Check sheet for the modelled part. Datum: model origin and axes. Units: mm. A direction names the side the tool comes from. Round coordinates to 2 decimals unless told otherwise and drop trailing zeros. Write each loop counter-clockwise with the first axis right and the second up, starting at its lowest first coordinate (ties: lowest second). Pieces come first, ordered by that corner, then holes. Notation, with made-up numbers: M 11.25,22 L 29.25,22 A18 ccw 29.25,53 Z; hole C 39.5,42 d10. An arc over 180 degrees is marked long. Answer in a Markdown table with one row per item.
```python
from build123d import *

# Parameters (mm, degrees)
SKETCH1_R           = 3.875
BOSS_EXTRUDE1_DEPTH = 29.78
SKETCH2_OUTSIDE_W   = 16.096
SKETCH2_OUTSIDE_H   = 16.096
SKETCH2_OUTSIDE_R   = 2.39
CUT_EXTRUDE1_DEPTH  = 25
CHAMFER1_SIZE       = 0.5
CUT_EXTRUDE2_DEPTH  = 3.36


with BuildPart() as part:
    # Sketch1 → Boss-Extrude1 (new body)
    with BuildSketch(Plane(origin=(0, 0, 0), x_dir=(1, 0, 0), z_dir=(0, 1, 0))):
        Circle(SKETCH1_R)
    extrude(amount=BOSS_EXTRUDE1_DEPTH)

    # Sketch2 outside → Cut-Extrude1 (cut)
    with BuildSketch(Plane(origin=(0, 29.78, 0), x_dir=(1, 0, 0), z_dir=(0, 1, 0))):
        Rectangle(SKETCH2_OUTSIDE_W, SKETCH2_OUTSIDE_H)
        Circle(SKETCH2_OUTSIDE_R, mode=Mode.SUBTRACT)
    extrude(amount=-CUT_EXTRUDE1_DEPTH, mode=Mode.SUBTRACT)

    # Chamfer1
    chamfer1_edges = [part.edges().sort_by_distance(p)[0] for p in [
        (-2.39, 29.78, 0),
    ]]
    chamfer(chamfer1_edges, length=CHAMFER1_SIZE)

    # Sketch8 → Cut-Extrude2 (cut)
    with BuildSketch(Plane.XZ):
        Polygon((2.644264233, 0), (1.322132116, 2.29), (-1.322132116, 2.29), (-2.644264233, 0), (-1.322132116, -2.29), (1.322132116, -2.29), align=None)
    extrude(amount=-CUT_EXTRUDE2_DEPTH, mode=Mode.SUBTRACT)


solid = part.part
```
1. Scan lines: L1, parallel to Y at x = -2.75, z = 0.25; L2, parallel to Z at x = 0, y = 14.25; L3, parallel to X at y = 2.5, z = 0.5. Record each from-to range of solid material in increasing order.
Found:
| item | result |
|---|---|
| L1 | y = 0 to 4.78 |
| L2 | z = -2.39 to 2.39 |
| L3 | x = -3.84 to -2.36, 2.36 to 3.84 |
2. Section check C-C, the plane z = 3.5. Record the cut outline in (x, y).
Found:
| item | result |
|---|---|
| outline | M -1.66,0 L 1.66,0 L 1.66,4.78 L -1.66,4.78 Z |
3. Access from +Z, -Z, +X, -X, +Y, -Y to the whole of each face (thin tool, end or side, straight path). Record for faces 1 (the face through (-2, 0, 2)), 2 (the face through (1.974, 1.656, -1.161)), 3 (the face through (-2, 4.78, 2)).
Found:
| item | result |
|---|---|
| face 1 | +Z, -Z, +X, -X, -Y |
| face 2 | -Y |
| face 3 | +Y |
4. Draft check along Z on faces 4 (the face through (0, 29.78, 0)), 5 (the face through (2.28, 17.2, -0.72)), 6 (the face through (0, 2, -2.29)). Enter one of: +Z half, -Z half, draft (parallel to the pull), parting line (faces both ways), or undercut.
Found:
| item | result |
|---|---|
| face 4 | draft |
| face 5 | parting line |
| face 6 | undercut |
5. Section check B-B, the plane y = 5.75. Record the cut outline in (x, z), and give its area (3 significant figures).
Found:
| item | result |
|---|---|
| outline | C 0,0 d4.78 |
| area | 17.9 mm2 |
6. Section check A-A, the plane x = 0. Record the cut outline in (y, z) (3 decimals).
Found:
| item | result |
|---|---|
| outline | M 0,-3.875 L 4.78,-3.875 L 4.78,-2.39 L 29.28,-2.39 L 29.78,-1.89 L 29.78,1.89 L 29.28,2.39 L 4.78,2.39 L 4.78,3.875 L 0,3.875 L 0,2.29 L 3.36,2.29 L 3.36,-2.29 L 0,-2.29 Z |
7. Go/stop test with flat-tipped pins: pin 1 (2 mm diameter, centred on x = 3, y = 26.5, fed in from +Z); pin 2 (1 mm diameter, centred on y = 22.5, z = -1, fed in from +X); pin 3 (4 mm diameter, centred on x = 2.5, y = 6.5, fed in from +Z). Record where each tip stops, or that it passes through.
Found:
| item | result |
|---|---|
| pin 1 | stops at z = 1.31 |
| pin 2 | stops at x = 2.34 |
| pin 3 | stops at z = 3.58 |
